```python
from build123d import *

# Parameters (mm, degrees)
F1_DEPTH = 3
F2_DEPTH = 1
F3_R     = 1
F3_2_R   = 1


# Not quite as in the source:
# - a feature names something its author has since deleted; it is built from what else it names


with BuildPart() as f1:
    # F0 (on Top) → F1 (new body)
    with BuildSketch(Plane.XY):
        with BuildLine():
            Line((-63.25, -34.2033516131), (-63.25, 26.5466483869))
            Line((-63.25, 26.5466483869), (-8.6602540378, 26.5466483869))
            ThreePointArc((-8.6602540378, 26.5466483869), (-9.6592582629, 28.9584579359), (-10, 31.5466483869))
            Line((-10, 31.5466483869), (-34.125, 31.5466483869))
            Line((-34.125, 31.5466483869), (-68.25, 31.5466483869))
            Line((-68.25, 31.5466483869), (-68.25, -36.7033516131))
            Line((-68.25, -36.7033516131), (0, -36.7033516131))
            Line((0, -36.7033516131), (0, 21.5466483869))
            ThreePointArc((0, 21.5466483869), (-1.2600429248, 21.6263514243), (-2.5, 21.8641900214))
            Line((-2.5, 21.8641900214), (-2.5, -34.2033516131))
            Line((-2.5, -34.2033516131), (-63.25, -34.2033516131))
        make_face()
        with BuildLine():
            ThreePointArc((-10, 31.5466483869), (-9.6592582629, 28.9584579359), (-8.6602540378, 26.5466483869))
            Line((-8.6602540378, 26.5466483869), (-5.4943754879, 26.5466483869))
            ThreePointArc((-5.4943754879, 26.5466483869), (-6.9283902407, 28.8660569086), (-7.4288735352, 31.5466483869))
            Line((-7.4288735352, 31.5466483869), (-10, 31.5466483869))
        make_face()
        with BuildLine():
            ThreePointArc((-7.4288735352, 31.5466483869), (-6.9283902407, 28.8660569086), (-5.4943754879, 26.5466483869))
            Line((-5.4943754879, 26.5466483869), (-2.5, 26.5466483869))
            Line((-2.5, 26.5466483869), (-2.5, 24.5510667812))
            ThreePointArc((-2.5, 24.5510667812), (-1.2686352802, 24.2268993115), (0, 24.1177748517))
            Line((0, 24.1177748517), (0, 31.5466483869))
            Line((0, 31.5466483869), (-7.4288735352, 31.5466483869))
        make_face()
        with BuildLine():
            ThreePointArc((0, 24.1177748517), (-1.2686352802, 24.2268993115), (-2.5, 24.5510667812))
            Line((-2.5, 24.5510667812), (-2.5, 21.8641900214))
            ThreePointArc((-2.5, 21.8641900214), (-1.2600429248, 21.6263514243), (0, 21.5466483869))
            Line((0, 21.5466483869), (0, 24.1177748517))
        make_face()
    extrude(amount=F1_DEPTH)

    # F0 (on Top) → F2 (join)
    with BuildSketch(Plane.XY):
        with BuildLine():
            Line((-8.6602540378, 26.5466483869), (-63.25, 26.5466483869))
            Line((-63.25, 26.5466483869), (-63.25, -34.2033516131))
            Line((-63.25, -34.2033516131), (-2.5, -34.2033516131))
            Line((-2.5, -34.2033516131), (-2.5, 21.8641900214))
            ThreePointArc((-2.5, 21.8641900214), (-3.5201478643, 22.1867039953), (-4.5, 22.6163628372))
            Line((-4.5, 22.6163628372), (-4.5, -32.2033516131))
            Line((-4.5, -32.2033516131), (-61.25, -32.2033516131))
            Line((-61.25, -32.2033516131), (-61.25, 24.5466483869))
            Line((-61.25, 24.5466483869), (-7.1414284285, 24.5466483869))
            ThreePointArc((-7.1414284285, 24.5466483869), (-7.9638741949, 25.4987803487), (-8.6602540378, 26.5466483869))
        make_face()
        with BuildLine():
            ThreePointArc((-10, 31.5466483869), (-9.6592582629, 28.9584579359), (-8.6602540378, 26.5466483869))
            Line((-8.6602540378, 26.5466483869), (-5.4943754879, 26.5466483869))
            ThreePointArc((-5.4943754879, 26.5466483869), (-6.9283902407, 28.8660569086), (-7.4288735352, 31.5466483869))
            Line((-7.4288735352, 31.5466483869), (-10, 31.5466483869))
        make_face()
        with BuildLine():
            Line((-5.4943754879, 26.5466483869), (-8.6602540378, 26.5466483869))
            ThreePointArc((-8.6602540378, 26.5466483869), (-7.9638741949, 25.4987803487), (-7.1414284285, 24.5466483869))
            Line((-7.1414284285, 24.5466483869), (-4.5, 24.5466483869))
            Line((-4.5, 24.5466483869), (-4.5, 22.6163628372))
            ThreePointArc((-4.5, 22.6163628372), (-3.5201478643, 22.1867039953), (-2.5, 21.8641900214))
            Line((-2.5, 21.8641900214), (-2.5, 24.5510667812))
            ThreePointArc((-2.5, 24.5510667812), (-4.1198417866, 25.364814868), (-5.4943754879, 26.5466483869))
        make_face()
        with BuildLine():
            Line((-2.5, 26.5466483869), (-5.4943754879, 26.5466483869))
            ThreePointArc((-5.4943754879, 26.5466483869), (-4.1198417866, 25.364814868), (-2.5, 24.5510667812))
            Line((-2.5, 24.5510667812), (-2.5, 26.5466483869))
        make_face()
    extrude(amount=F2_DEPTH)

    # F3
    f3_edges = [f1.edges().sort_by_distance(p)[0] for p in [
        (-32.875, 26.546648, 3),
        (-63.25, -3.828352, 3),
        (-32.875, -34.203352, 3),
        (-2.5, -3.828352, 3),
        (-34.125, 31.546648, 3),
        (-68.25, -2.578352, 3),
    ]]
    fillet(f3_edges, radius=F3_R)



with BuildPart() as f1b:
    # F0 (on Top) → F1, piece 2 (new body)
    with BuildSketch(Plane.XY):
        with BuildLine():
            ThreePointArc((8.6602540378, 26.5466483869), (9.6592582629, 28.9584579359), (10, 31.5466483869))
            Line((10, 31.5466483869), (7.4288735352, 31.5466483869))
            ThreePointArc((7.4288735352, 31.5466483869), (6.9283902407, 28.8660569086), (5.4943754879, 26.5466483869))
            Line((5.4943754879, 26.5466483869), (8.6602540378, 26.5466483869))
        make_face()
    extrude(amount=F1_DEPTH)

    # F0 (on Top) → F2, piece 2 (join)
    with BuildSketch(Plane.XY):
        with BuildLine():
            ThreePointArc((8.6602540378, 26.5466483869), (9.6592582629, 28.9584579359), (10, 31.5466483869))
            Line((10, 31.5466483869), (7.4288735352, 31.5466483869))
            ThreePointArc((7.4288735352, 31.5466483869), (6.9283902407, 28.8660569086), (5.4943754879, 26.5466483869))
            Line((5.4943754879, 26.5466483869), (8.6602540378, 26.5466483869))
        make_face()
    extrude(amount=F2_DEPTH)

    # F3#2
    f3_2_edges = [f1b.edges().sort_by_distance(p)[0] for p in [
        (9.659258, 28.958458, 3),
        (6.92839, 28.866057, 3),
        (7.077315, 26.546648, 3),
        (8.714437, 31.546648, 3),
    ]]
    fillet(f3_2_edges, radius=F3_2_R)


with BuildPart() as f1_1:
    add(f1.part)

    add(f1b.part)  # F4 merges F1b
    # F4: F1 across plane
    add(f1.part.mirror(Plane.YZ))

    # F5: F1 across face


with BuildPart() as f1_2:
    add(f1_1.part)
    add(f1_1.part.mirror(Plane(origin=(0, -36.7033516131, 1.4986605371), x_dir=(1, 0, 0), z_dir=(0, -1, 0))))


solid = f1_2.part
```
Source: CAD feature listing. Evaluate the final solid. Frame: model axes, mm. A direction names the side the tool comes from. Round coordinates to 2 decimals unless told otherwise and drop trailing zeros. Order: outer loops, then holes, each group sorted by start corner. A loop starts at its lowest first (then second) coordinate and runs counter-clockwise, first axis right, second up. Notation, with made-up numbers: (53.5, 89) -> (92.5, 89) arc R27 cw to (92.5, 124) -> close; hole circle Ø2 at (37, 25). An arc over 180 degrees is marked (long way). Use CSV: the item, a comma, the result in double quotes.
(1) Section A-A on y = -0.5. Return the cut outline in (x, z), and give its area (3 significant figures).
Report:
outline,"(-68.25, 0) -> (-61.25, 0) -> (-61.25, 1) -> (-63.25, 1) -> (-63.25, 2) arc R1 ccw to (-64.25, 3) -> (-67.25, 3) arc R1 ccw to (-68.25, 2) -> close; (-4.5, 0) -> (4.5, 0) -> (4.5, 1) -> (2.5, 1) -> (2.5, 2) arc R1 ccw to (1.5, 3) -> (-1.5, 3) arc R1 ccw to (-2.5, 2) -> (-2.5, 1) -> (-4.5, 1) -> close; (61.25, 0) -> (68.25, 0) -> (68.25, 2) arc R1 ccw to (67.25, 3) -> (64.25, 3) arc R1 ccw to (63.25, 2) -> (63.25, 1) -> (61.25, 1) -> close"
area,"51.7 mm^2"
(2) Ray query, L1, parallel to Y at x = -61, z = 0.95; L2, parallel to X at y = 7, z = 1.7; L3, parallel to Y at x = -21.5, z = 2.2. Return the intervals inside material, ascending.
Report:
L1,"-104.95 to -97.95, -41.2 to -32.2, 24.55 to 31.55"
L2,"-68.25 to -63.25, -2.5 to 2.5, 63.25 to 68.25"
L3,"-104.93 to -99.97, -39.18 to -34.22, 26.57 to 31.53"
(3) Access query for faces 3 (the face through (-35, -40, 1)), 4 (the face through (16, -38, 0)). Directions: +Z, -Z, +X, -X, +Y, -Y. A direction counts if a zero-diameter tool reaches every point of the face in a straight line with its end or side. Return the directions, or none.
Report:
face 3,"+Z"
face 4,"-Z, +X, -X, +Y, -Y"
(4) Pull-direction query (Y, two-part tool) for faces 1 (the face through (-35, -33, 1)), 2 (the face through (0, -37, 3)); classes: +Y half, -Y half, draft (parallel to the pull), parting line (faces both ways), or undercut.
Report:
face 1,"undercut"
face 2,"draft"
(5) Section B-B on x = -24. Return the cut outline in (y, z).
Report:
outline,"(-104.95, 0) -> (-97.95, 0) -> (-97.95, 1) -> (-99.95, 1) -> (-99.95, 2) arc R1 ccw to (-100.95, 3) -> (-103.95, 3) arc R1 ccw to (-104.95, 2) -> close; (-41.2, 0) -> (-32.2, 0) -> (-32.2, 1) -> (-34.2, 1) -> (-34.2, 2) arc R1 ccw to (-35.2, 3) -> (-38.2, 3) arc R1 ccw to (-39.2, 2) -> (-39.2, 1) -> (-41.2, 1) -> close; (24.55, 0) -> (31.55, 0) -> (31.55, 2) arc R1 ccw to (30.55, 3) -> (27.55, 3) arc R1 ccw to (26.55, 2) -> (26.55, 1) -> (24.55, 1) -> close"
